Part model, mm, in its own coordinate system. Face numbers are marked on the shaded views. A direction names the side the tool comes from. Round coordinates to 2 decimals unless told otherwise and drop trailing zeros. Loops run counter-clockwise (first coordinate to the right, second up) from the corner with the lowest first, then second, coordinate; pieces in that order, holes last.
(1) Cut at D-D on x = 5.5. List the corners of the cut face in (y, z).
(2) Cut at C-C on z = 3.9. Count the separate pieces of the cut face and the enclosed holes in it, then the cut area to 3 significant figures.
(3) Tool access for the marked faces 1 and 2: list every direction of +Z, -Z, +X, -X, +Y, -Y with a clear straight run to the whole face (end or side of a thin tool).
(4) Cut at B-B on y = -5. List the corners of the cut face in (x, z).
(5) Cut at A-A on x = 0. List the corners of the cut face in (y, z).
(6) Probe probe 1 along X at (y, z) = (1.25, 4.75); probe 2 along Y at (x, z) = (-6.5, 1.7); probe 3 along Y at (x, z) = (-5, 1.05). List the from-to ranges inside material, lowest first.
(7) Flat gauge pins, fed straight in: pin 1 (3 mm diameter, centred on y = 3, z = 2.5, fed in from -X); pin 2 (3 mm diameter, centred on y = 9, z = 5, fed in from +X); pin 3 (1 mm diameter, centred on y = 7.5, z = 2.5, fed in from -X). Where does each tip first touch, or does it go through?
(8) Mould opens along Y. For the marked faces 3, 4 and 5 say: +Y half, -Y half, draft (parallel to the pull), parting line (faces both ways), or undercut.
from build123d import *

# Parameters (mm, degrees)
SKETCH_1_R      = 14
EXTRUDE_1_DEPTH = 6


with BuildPart() as part:
    # 草图1 → 凸台-拉伸1 (new body)
    with BuildSketch(Plane.XY):
        Circle(SKETCH_1_R)
        with BuildLine():
            Line((4.596960215, -1.205253518), (9.199687971, -3.477076493))
            ThreePointArc((9.199687971, -3.477076493), (9.69373922, -3.490261664), (10.024736471, -3.123244898))
            ThreePointArc((10.024736471, -3.123244898), (9.09326674, 5.25), (2.307558811, 10.243298899))
            ThreePointArc((2.307558811, 10.243298899), (1.824214343, 10.140155255), (1.588607412, 9.705701736))
            Line((1.588607412, 9.705701736), (1.254699943, 4.583711086))
            ThreePointArc((1.254699943, 4.583711086), (1.392222532, 3.981727051), (1.836894199, 3.553282947))
            ThreePointArc((1.836894199, 3.553282947), (3.464101615, 2), (3.995680398, -0.185844433))
            ThreePointArc((3.995680398, -0.185844433), (4.144388043, -0.785163445), (4.596960215, -1.205253518))
        make_face(mode=Mode.SUBTRACT)
        with BuildLine():
            Line((-1.254699943, 4.583711086), (-1.588607412, 9.705701736))
            ThreePointArc((-1.588607412, 9.705701736), (-1.824214343, 10.140155255), (-2.307558811, 10.243298899))
            ThreePointArc((-2.307558811, 10.243298899), (-9.09326674, 5.25), (-10.024736471, -3.123244898))
            ThreePointArc((-10.024736471, -3.123244898), (-9.69373922, -3.490261664), (-9.199687971, -3.477076493))
            Line((-9.199687971, -3.477076493), (-4.596960215, -1.205253518))
            ThreePointArc((-4.596960215, -1.205253518), (-4.144388043, -0.785163445), (-3.995680398, -0.185844433))
            ThreePointArc((-3.995680398, -0.185844433), (-3.919805533, 0.79694704), (-3.605891638, 1.731342108))
            Line((-3.605891638, 1.731342108), (-1.423938852, 0.471591079))
            ThreePointArc((-1.423938852, 0.471591079), (-1.061904855, -1.059414026), (0.468245837, -1.425042398))
            Line((0.468245837, -1.425042398), (1.468245837, 0.307008409))
            ThreePointArc((1.468245837, 0.307008409), (0.386527032, 1.449343594), (-1.120379281, 0.99737168))
            Line((-1.120379281, 0.99737168), (-3.302332067, 2.257122708))
            ThreePointArc((-3.302332067, 2.257122708), (-2.650079149, 2.996177649), (-1.836894199, 3.553282947))
            ThreePointArc((-1.836894199, 3.553282947), (-1.392222532, 3.981727051), (-1.254699943, 4.583711086))
        make_face(mode=Mode.SUBTRACT)
        with BuildLine():
            Line((3.342260273, -3.378457568), (7.611080559, -6.228625243))
            ThreePointArc((7.611080559, -6.228625243), (7.869524877, -6.649893591), (7.717177659, -7.120054001))
            ThreePointArc((7.717177659, -7.120054001), (0, -10.5), (-7.717177659, -7.120054001))
            ThreePointArc((-7.717177659, -7.120054001), (-7.869524877, -6.649893591), (-7.611080559, -6.228625243))
            Line((-7.611080559, -6.228625243), (-3.342260273, -3.378457568))
            ThreePointArc((-3.342260273, -3.378457568), (-2.752165511, -3.196563606), (-2.1587862, -3.367438514))
            ThreePointArc((-2.1587862, -3.367438514), (0, -4), (2.1587862, -3.367438514))
            ThreePointArc((2.1587862, -3.367438514), (2.752165511, -3.196563606), (3.342260273, -3.378457568))
        make_face(mode=Mode.SUBTRACT)
    extrude(amount=EXTRUDE_1_DEPTH)


solid = part.part
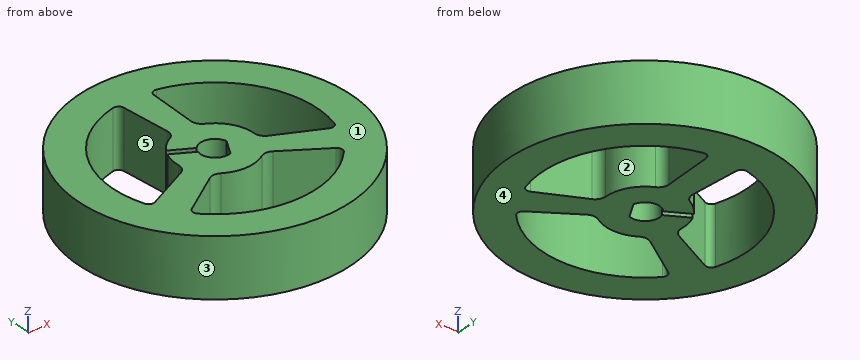
Final values:
1. outline: (-12.87, 0) - (-8.94, 0) - (-8.94, 6) - (-12.87, 6) - close; (-4.82, 0) - (-1.65, 0) - (-1.65, 6) - (-4.82, 6) - close; (8.94, 0) - (12.87, 0) - (12.87, 6) - (8.94, 6) - close
2. separate pieces: 1
2. enclosed holes: 3
2. area: 369 mm2
3. face 1: +Z, +X, -X, +Y, -Y
3. face 2: +Z, -Z
4. outline: (-13.08, 0) - (-5.77, 0) - (-5.77, 6) - (-13.08, 6) - close; (5.77, 0) - (13.08, 0) - (13.08, 6) - (5.77, 6) - close
5. outline: (-14, 0) - (-10.5, 0) - (-10.5, 6) - (-14, 6) - close; (-4, 0) - (-1.5, 0) - (-1.5, 6) - (-4, 6) - close; (1.5, 0) - (14, 0) - (14, 6) - (1.5, 6) - close
6. probe 1: x = -13.94 to -10.43, -3.8 to -2.77, -1.56 to -0.83, 0.83 to 3.8, 10.43 to 13.94
6. probe 2: y = -12.4 to -8.25, -5.49 to -2.14, 8.25 to 12.4
6. probe 3: y = -13.08 to -9.23, -4.49 to -1.4, 9.23 to 13.08
7. pin 1: stops at x = -13.92
7. pin 2: stops at x = 11.82
7. pin 3: stops at x = -12.12
8. face 3: parting line
8. face 4: draft
8. face 5: undercut
